from build123d import *

# Parameters (mm, degrees)
F0_W     = 57.15
F0_H     = 50.8
F1_DEPTH = 88.9
F2_W     = 24.023754
F2_H     = 20.589164
F3_DEPTH = 85.725
F2_W_2   = 23.884728
F2_H_2   = 20.685836
F4_DEPTH = 85.725
F2_W_3   = 23.601246
F2_H_3   = 20.868859
F5_DEPTH = 85.725
F2_W_4   = 23.534088
F2_H_4   = 20.412843
F6_DEPTH = 85.725


with BuildPart() as f1:
    # F0 (on Top) → F1 (new body)
    with BuildSketch(Plane.XY):
        Rectangle(F0_W, F0_H)
    extrude(amount=F1_DEPTH)

    # F2 (on face) → F3 (cut)
    with BuildSketch(Plane.XY.offset(88.9)):
        with Locations((-13.388123, 11.930418)):
            Rectangle(F2_W, F2_H)
    extrude(amount=-F3_DEPTH, mode=Mode.SUBTRACT)

    # F2 (on face) → F4 (cut)
    with BuildSketch(Plane.XY.offset(88.9)):
        with Locations((-13.457636, -11.882082)):
            Rectangle(F2_W_2, F2_H_2)
    extrude(amount=-F4_DEPTH, mode=Mode.SUBTRACT)

    # F2 (on face) → F5 (cut)
    with BuildSketch(Plane.XY.offset(88.9)):
        with Locations((13.599377, 11.79057)):
            Rectangle(F2_W_3, F2_H_3)
    extrude(amount=-F5_DEPTH, mode=Mode.SUBTRACT)

    # F2 (on face) → F6 (cut)
    with BuildSketch(Plane.XY.offset(88.9)):
        with Locations((13.426772, -12.018578)):
            Rectangle(F2_W_4, F2_H_4)
    extrude(amount=-F6_DEPTH, mode=Mode.SUBTRACT)


solid = f1.part
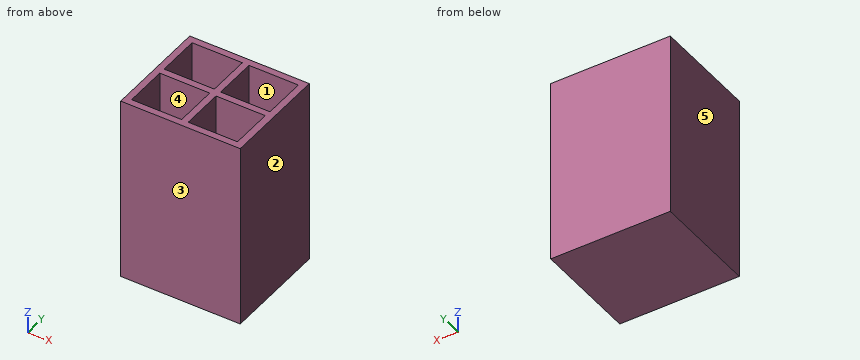
For this review, take the finished solid that the model builds, in its own axes (mm). Face numbers are marked on the shaded views. A direction names the side the tool comes from. Give positions to 0.01 mm unless a question says otherwise; leave off trailing zeros. Order: outer loops, then holes, each group sorted by start corner. A loop starts at its lowest first (then second) coordinate and runs counter-clockwise, first axis right, second up. Notation, with made-up numbers: (14, 28) - (20, 28) arc R22 cw to (20, 54) - close; hole circle Ø4 at (-4, 5). An arc over 180 degrees is marked (long way). Answer as a JSON object with one key per item and string values. Group by question number.
Item 1: Take a section at B-B on y = 11.5. Give the boundary of the cut face in (x, z) (3 decimals), and give its area (3 significant figures).
Item 2: Clearance check with a flat-ended pin moving along its axis: pin 1 Ø16.5 at (x, y) = (-15.5, 10) entering from +Z (3 decimals). State where the tip first meets the part, or that it passes through.
Item 3: Draft analysis for pull direction Y (two halves, no side actions). For the marked faces 1, 2 and 3, state which applies: pulls with the +Y half, pulls with the -Y half, needs draft (parallel to the pull), parting line crosses it, or undercut.
Item 4: Take a section at A-A on x = -23. Give the boundary of the cut face in (y, z) (3 decimals).
Item 5: Machinability: for the marked faces 4 and 5, which of the approach directions +Z, -Z, +X, -X, +Y, -Y give a long, thin tool a straight path to every point of the face, cutting with its end or side? Answer none if there is none.
Item 6: Take a section at C-C on z = 15.5. Give the boundary of the cut face in (x, y) (3 decimals).
Item 7: Wall thickness on line 1 along X through (y, z) = (-8, 9.5) (3 decimals); line 2 along X through (y, z) = (7.5, 8.5) (3 decimals); line 3 along Y through (x, z) = (14, 38) (3 decimals): over which ranges is each line inside the solid? List them lowest first.
Reported:
{
 "1": {"outline": "(-28.575, 0) - (28.575, 0) - (28.575, 88.9) - (25.4, 88.9) - (25.4, 3.175) - (1.799, 3.175) - (1.799, 88.9) - (-1.376, 88.9) - (-1.376, 3.175) - (-25.4, 3.175) - (-25.4, 88.9) - (-28.575, 88.9) - close", "area": "998 mm^2"},
 "2": {"pin 1": "z = 3.175"},
 "3": {"face 1": "undercut", "face 2": "needs draft", "face 3": "pulls with the -Y half"},
 "4": {"outline": "(-25.4, 0) - (25.4, 0) - (25.4, 88.9) - (22.225, 88.9) - (22.225, 3.175) - (1.636, 3.175) - (1.636, 88.9) - (-1.539, 88.9) - (-1.539, 3.175) - (-22.225, 3.175) - (-22.225, 88.9) - (-25.4, 88.9) - close"},
 "5": {"face 4": "+Z", "face 5": "+Z, -Z, -X, +Y, -Y"},
 "6": {"outline": "(-28.575, -25.4) - (28.575, -25.4) - (28.575, 25.4) - (-28.575, 25.4) - close; hole (-25.4, -22.225) - (-1.515, -22.225) - (-1.515, -1.539) - (-25.4, -1.539) - close; hole (-25.4, 1.636) - (-1.376, 1.636) - (-1.376, 22.225) - (-25.4, 22.225) - close; hole (1.66, -22.225) - (25.194, -22.225) - (25.194, -1.812) - (1.66, -1.812) - close; hole (1.799, 1.356) - (25.4, 1.356) - (25.4, 22.225) - (1.799, 22.225) - close"},
 "7": {"line 1": "-28.575 to -25.4, -1.515 to 1.66, 25.194 to 28.575", "line 2": "-28.575 to -25.4, -1.376 to 1.799, 25.4 to 28.575", "line 3": "-25.4 to -22.225, -1.812 to 1.356, 22.225 to 25.4"}
}
